Could you check a few things on this model? Use its own coordinates, in mm. Face numbers are marked on the shaded views. A direction names the side the tool comes from. Coordinates: 2 decimals unless noted, no trailing zeros. Loops run counter-clockwise (first coordinate to the right, second up) from the corner with the lowest first, then second, coordinate; pieces in that order, holes last.
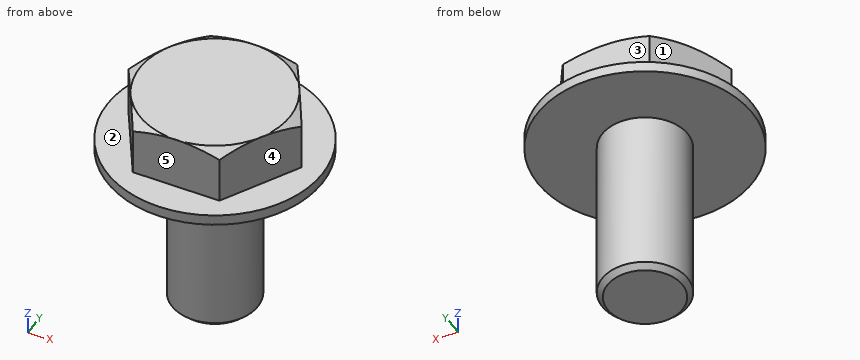
Solid Edge part; units mm, degrees
sketch "Sketch1" plane through (0, 0, 0) normal (0, 0, 1) x (1, 0, 0)
  circle A0 centre (0, 0) radius 5
extrude "Protrusion1" add sketch "Sketch1" against normal blind 0.5
sketch "Sketch2" plane through (0, 0, 0) normal (0, 0, 1) x (1, 0, 0)
  line L0 (2.0207, 3.5) -> (-2.0207, 3.5)
  line L1 (-2.0207, 3.5) -> (-4.0415, 0)
  line L2 (-4.0415, 0) -> (-2.0207, -3.5)
  line L3 (-2.0207, -3.5) -> (2.0207, -3.5)
  line L4 (2.0207, -3.5) -> (4.0415, 0)
  line L5 (4.0415, 0) -> (2.0207, 3.5)
extrude "Protrusion2" add sketch "Sketch2" along normal blind 2.5
sketch "Sketch3" plane through (0, 0, 0) normal (1, 0, 0) x (0, 1, 0)
  line L0 (-3.495, 2.5) -> (-6.9591, 0.5)
revolve "RevolvedCutout1" cut sketch "Sketch3" angle 360 about axis through (0, 0, 2.5) along (0, 0, -1) material side at (0, -5.2521, 1.5433)
sketch "Sketch4" plane through (0, 0, -0.5) normal (0, 0, -1) x (0, 1, 0)
  circle A0 centre (0, 0) radius 2
extrude "Protrusion3" add sketch "Sketch4" along normal blind 8
chamfer "Chamfer1" distance 0.25 angle 45 1 edges at (0, -2, -8.5)
properties part number "BOLT1" material "Steel"
1) Imagine slicing it at A-A on x = 0. List the corners of the cut face in (y, z) for me (3 decimals), plus the area to 3 significant figures.
2) For the marked faces 1, 2, 3, 4 and 5, which set-ups out of +Z, -Z, +X, -X, +Y, -Y let a thin tool reach every point of the face, with its end or its side?
3) Imagine slicing it at D-D on x = 4.75. List the corners of the cut face in (y, z) for me, plus the area to 3 significant figures.
4) Imagine slicing it at C-C on z = -1.5. List the corners of the cut face in (x, y) for me.
5) If I drill on L1, parallel to Y at x = 1.5, z = 1; L2, parallel to Z at x = -1.5, y = 4.25; L3, parallel to Z at x = 0.25, y = -2.25, over which ranges is the centre line in solid material (lowest first)?
6) Imagine slicing it at B-B on z = 0.75. List the corners of the cut face in (x, y) for me.
7) Will these pins go through, and if not, where does the flat tip stop? pin 1 (2 mm diameter, centred on x = 3.5, z = -1, fed in from +Y); pin 2 (1.5 mm diameter, centred on x = -3.5, y = -2, fed in from +Z); pin 3 (2 mm diameter, centred on x = 1.5, z = -1, fed in from +Y); pin 4 (2 mm diameter, centred on x = 0, z = 2, fed in from -Y).
Solved:
1. outline: (-5, -0.5) - (-2, -0.5) - (-2, -8.25) - (-1.75, -8.5) - (1.75, -8.5) - (2, -8.25) - (2, -0.5) - (5, -0.5) - (5, 0) - (3.5, 0) - (3.5, 2.497) - (3.495, 2.5) - (-3.495, 2.5) - (-3.5, 2.497) - (-3.5, 0) - (-5, 0) - close
1. area: 54.4 mm2
2. face 1: +Z, -X, +Y
2. face 2: +Z
2. face 3: +Z, +X, -X, +Y
2. face 4: +Z, +X, -Y
2. face 5: +Z, +X, -X, -Y
3. outline: (-1.56, -0.5) - (1.56, -0.5) - (1.56, 0) - (-1.56, 0) - close
3. area: 1.56 mm2
4. outline: circle Ø4 at (0, 0)
5. L1: y = -3.5 to 3.5
5. L2: z = -0.5 to 0
5. L3: z = -0.5 to 2.5
6. outline: (-4.04, 0) - (-2.02, -3.5) - (2.02, -3.5) - (4.04, 0) - (2.02, 3.5) - (-2.02, 3.5) - close
7. pin 1: stops at y = 4.25
7. pin 2: stops at z = 2.5
7. pin 3: stops at y = 4.96
7. pin 4: stops at y = -3.5
